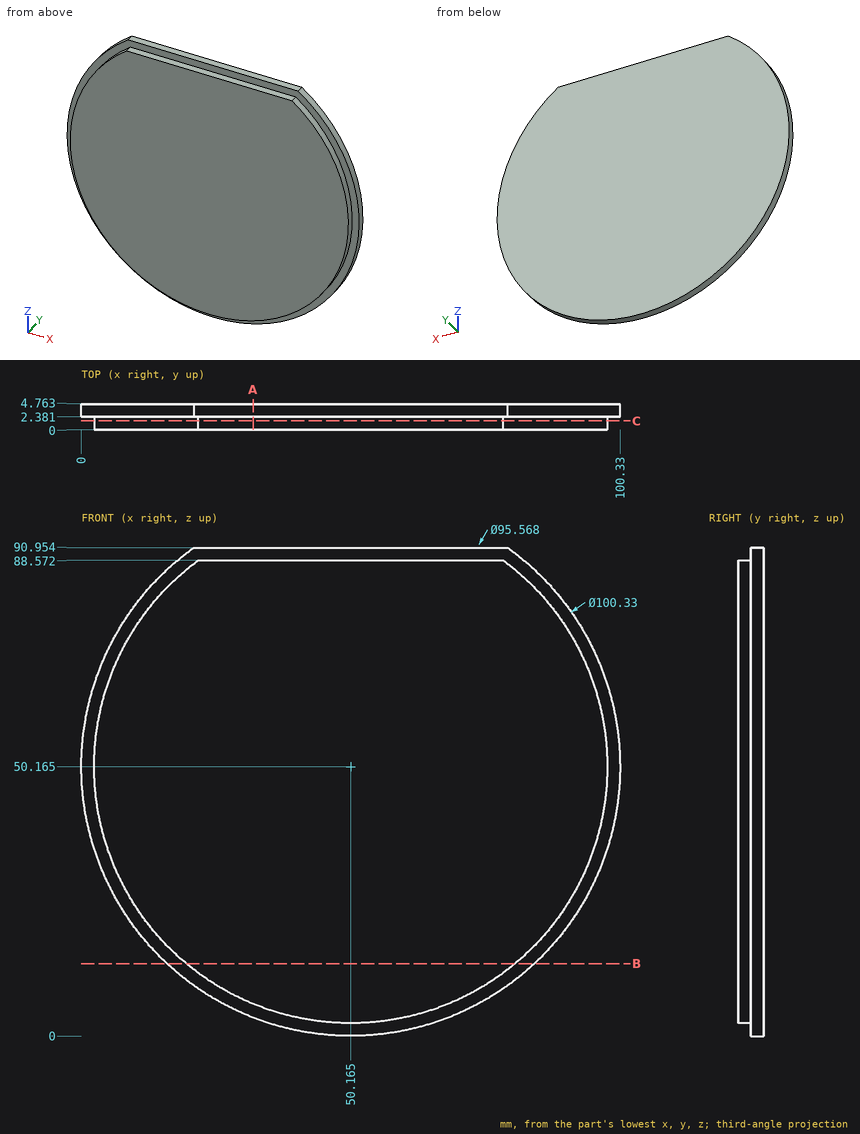
Geometry: see drawing. Coordinates: mm, zero at the bounding-box minimum. Round coordinates to 2 decimals unless told otherwise and drop trailing zeros. Loops run counter-clockwise (first coordinate to the right, second up) from the corner with the lowest first, then second, coordinate; pieces in that order, holes last. Notation, with made-up numbers: M 83,-21 L 95,-21 A19 ccw 95,12 Z; hole C 63.5,-34.5 d6. An arc over 180 degrees is marked long. Use a Markdown table: item, result. Add a question column.
1. Section query C-C on y = 1.6. Return the cut outline in (x, z) (1 decimal), then the cut area to 3 significant figures.
2. Section query B-B on z = 13.5. Return the cut outline in (x, y), then the cut area to 3 significant figures.
3. Contact query for a flat-ended pin moving along its axis: P1, Ø2.5, axis at x = 51.5, y = 1.5, coming from the +Z side. Output: stop coordinate, or through.
4. Section query A-A on x = 32. Return the cut outline in (y, z) (1 decimal).
5. Line query: line 1 (X direction, y = 2, z = 49.5) (1 decimal); line 2 (Y direction, x = 19, z = 87); line 3 (X direction, y = 1.2, z = 15) (1 decimal). Output: solid intervals per line, ascending.
Reported:
| question | item | result |
|---|---|---|
| 1 | outline | M 21.7,88.6 A47.8 ccw long 78.6,88.6 Z |
| 1 | area | 6,810 mm² |
| 2 | outline | M 15.93,2.38 L 19.52,2.38 L 19.52,0 L 80.81,0 L 80.81,2.38 L 84.4,2.38 L 84.4,4.76 L 15.93,4.76 Z |
| 2 | area | 309 mm² |
| 3 | P1 | stops at z = 90.95 |
| 4 | outline | M 0,6 L 2.4,6 L 2.4,3.4 L 4.8,3.4 L 4.8,91 L 2.4,91 L 2.4,88.6 L 0,88.6 Z |
| 5 | line 1 | x = 2.4 to 97.9 |
| 5 | line 2 | y = 2.38 to 4.76 |
| 5 | line 3 | x = 17.8 to 82.5 |
